Geometry check sheet. Reference: the model listing, model coordinates, mm. Face numbers are marked on the shaded views. A direction names the side the tool comes from. Coordinates: 2 decimals unless noted, no trailing zeros. Write each loop counter-clockwise with the first axis right and the second up, starting at its lowest first coordinate (ties: lowest second). Pieces come first, ordered by that corner, then holes. Notation, with made-up numbers: M 57.25,59.5 L 106.25,59.5 A25 cw 106.25,87.5 Z; hole C -0.5,-32.5 d1. An arc over 180 degrees is marked long. Put each result on its own line as item: value. Start each with the question number.
1) Scan lines: line 1 along X through (y, z) = (5.25, 0); line 2 along X through (y, z) = (2.25, 4.5); line 3 along Y through (x, z) = (0, 9.5). Record each from-to range of solid material in increasing order.
2) Cross-section at B-B on x = 0. Record the cut outline in (y, z), plus the area to 3 significant figures.
3) Cross-section at A-A on z = 0. Record the cut outline in (x, y), plus the area to 3 significant figures.
4) Set-up check for the marked faces 1 and 2: record each of +Z, -Z, +X, -X, +Y, -Y from which the full face is reachable in a straight line by a thin tool's end or side.
5) Cross-section at C-C on y = 1. Record the cut outline in (x, z), plus the area to 3 significant figures.
6) Cross-section at D-D on z = 5.08. Record the cut outline in (x, y) (3 decimals).
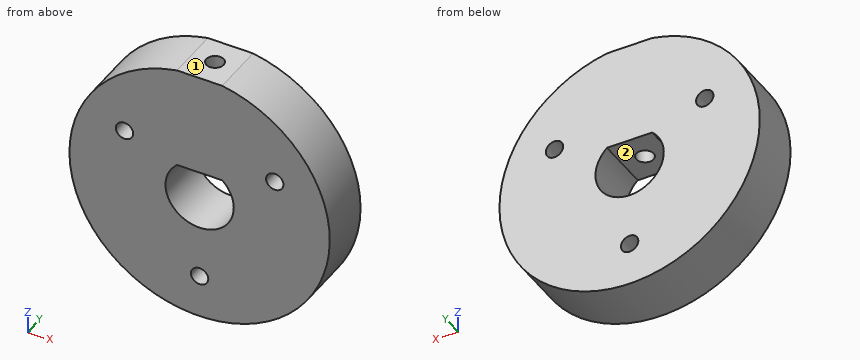
from build123d import *

# Parameters (mm, degrees)
SKETCH1_R           = 1.016
BOSS_EXTRUDE1_DEPTH = 6.35
CUT_EXTRUDE1_REACH  = 32.249
SKETCH2_R           = 1.016


with BuildPart() as part:
    # Sketch1 → Boss-Extrude1 (new body)
    with BuildSketch(Plane(origin=(0, 0, 0), x_dir=(1, 0, 0), z_dir=(0, 1, 0))):
        with BuildLine():
            Line((-2.645751311, -15.00858421), (2.645751311, -15.00858421))
            ThreePointArc((2.645751311, -15.00858421), (0, 15.24), (-2.645751311, -15.00858421))
        make_face()
        with Locations((0, 10.16)):
            Circle(SKETCH1_R, mode=Mode.SUBTRACT)
        with Locations((8.798818102, -5.08)):
            Circle(SKETCH1_R, mode=Mode.SUBTRACT)
        with Locations((-8.798818102, -5.08)):
            Circle(SKETCH1_R, mode=Mode.SUBTRACT)
        with BuildLine():
            Line((-2.645751311, -3), (2.645751311, -3))
            ThreePointArc((2.645751311, -3), (0, 4), (-2.645751311, -3))
        make_face(mode=Mode.SUBTRACT)
    extrude(amount=BOSS_EXTRUDE1_DEPTH)

    # Sketch2 → Cut-Extrude1 (cut, up to next)
    with BuildSketch(Plane.XY.offset(15.00858421), mode=Mode.PRIVATE) as cut_extrude1_sk1:
        with Locations((0, 3.175)):
            Circle(SKETCH2_R)
    cut_extrude1_tool1 = extrude(cut_extrude1_sk1.sketch, amount=-CUT_EXTRUDE1_REACH, mode=Mode.PRIVATE) & part.part
    add(cut_extrude1_tool1.solids().sort_by_distance((0, 3.175, 15.008584))[0], mode=Mode.SUBTRACT)


solid = part.part
Answer key:
1. line 1: x = -15.24 to -4, 4 to 15.24
1. line 2: x = -14.56 to -9.63, -7.96 to -0.42, 0.42 to 7.96, 9.63 to 14.56
1. line 3: y = 0 to 2.16, 4.19 to 6.35
2. outline: M 0,-15.24 L 6.35,-15.24 L 6.35,-11.18 L 0,-11.18 Z; M 0,-9.14 L 6.35,-9.14 L 6.35,-4 L 0,-4 Z; M 0,3 L 2.16,3 L 2.16,15.01 L 0,15.01 Z; M 4.19,3 L 6.35,3 L 6.35,15.01 L 4.19,15.01 Z
2. area: 110 mm²
3. outline: M -15.24,0 L -4,0 L -4,6.35 L -15.24,6.35 Z; M 4,0 L 15.24,0 L 15.24,6.35 L 4,6.35 Z
3. area: 143 mm²
4. face 1: +Z, +X, -X, +Y, -Y
4. face 2: +Y, -Y
5. outline: M -2.65,15.01 A15.24 ccw long 2.65,15.01 Z; hole C -8.8,5.08 d2.03; hole M -2.65,3 A4 ccw long 2.65,3 Z; hole C 0,-10.16 d2.03; hole C 8.8,5.08 d2.03
5. area: 672 mm²
6. outline: M -14.368,0 L -9.815,0 L -9.815,6.35 L -14.368,6.35 Z; M -7.783,0 L 7.783,0 L 7.783,6.35 L -7.783,6.35 Z; M 9.815,0 L 14.368,0 L 14.368,6.35 L 9.815,6.35 Z; hole C 0,3.175 d2.032
